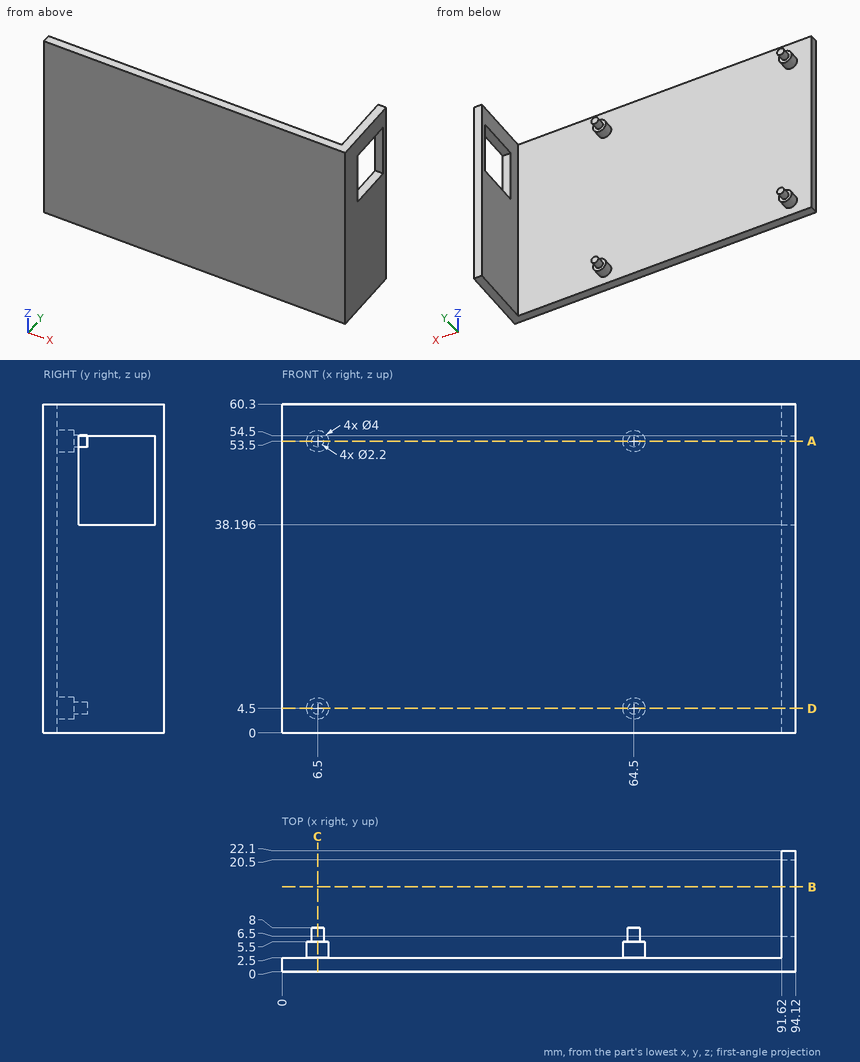
Geometry check sheet. Reference: drawing and pictorial views, mm from the part's lowest x, y, z. Coordinates: 2 decimals unless noted, no trailing zeros. Order: outer loops, then holes, each group sorted by start corner. A loop starts at its lowest first (then second) coordinate and runs counter-clockwise, first axis right, second up. Notation, with made-up numbers: (27, 78.5) - (42, 78.5) arc R18 ccw to (42, 98.5) - close; hole circle Ø8 at (73.5, -20.5). An arc over 180 degrees is marked (long way). Answer in a Markdown table with one row per item. Add a question column.
1) Cross-section at C-C, the plane x = 6.5. Record the cut outline in (y, z).
2) Material ranges on line 1 along Y through (x, z) = (12, 9.5); line 2 along X through (y, z) = (10.5, 20), recorded low to high. Write a range as [from, to].
3) Cross-section at D-D, the plane z = 4.5. Record the cut outline in (x, y).
4) Cross-section at B-B, the plane y = 15.5. Record the cut outline in (x, z), then the cut area to 3 significant figures.
5) Gauge pin test, flat ends, axial feed: P1, Ø6, axis at x = 52, z = 25.5, coming from the +Y side; P2, Ø1.8, axis at x = 64, z = 4.5, coming from the +Y side. Record the tip position at first contact, or that the pin passes through.
6) Cross-section at A-A, the plane z = 53.5. Record the cut outline in (x, y), then the cut area to 3 significant figures.
Check result:
| question | item | result |
|---|---|---|
| 1 | outline | (0, 0) - (2.5, 0) - (2.5, 2.5) - (5.5, 2.5) - (5.5, 3.4) - (8, 3.4) - (8, 5.6) - (5.5, 5.6) - (5.5, 6.5) - (2.5, 6.5) - (2.5, 51.5) - (5.5, 51.5) - (5.5, 52.4) - (8, 52.4) - (8, 54.6) - (5.5, 54.6) - (5.5, 55.5) - (2.5, 55.5) - (2.5, 60.3) - (0, 60.3) - close |
| 2 | line 1 | y = [0, 2.5] |
| 2 | line 2 | x = [91.62, 94.12] |
| 3 | outline | (0, 0) - (94.12, 0) - (94.12, 22.1) - (91.62, 22.1) - (91.62, 2.5) - (66.5, 2.5) - (66.5, 5.5) - (65.6, 5.5) - (65.6, 8) - (63.4, 8) - (63.4, 5.5) - (62.5, 5.5) - (62.5, 2.5) - (8.5, 2.5) - (8.5, 5.5) - (7.6, 5.5) - (7.6, 8) - (5.4, 8) - (5.4, 5.5) - (4.5, 5.5) - (4.5, 2.5) - (0, 2.5) - close |
| 4 | outline | (91.62, 0) - (94.12, 0) - (94.12, 38.2) - (91.62, 38.2) - close; (91.62, 54.5) - (94.12, 54.5) - (94.12, 60.3) - (91.62, 60.3) - close |
| 4 | area | 110 mm² |
| 5 | P1 | stops at y = 2.5 |
| 5 | P2 | stops at y = 8 |
| 6 | outline | (0, 0) - (94.12, 0) - (94.12, 6.5) - (91.62, 6.5) - (91.62, 2.5) - (66.5, 2.5) - (66.5, 5.5) - (65.6, 5.5) - (65.6, 8) - (63.4, 8) - (63.4, 5.5) - (62.5, 5.5) - (62.5, 2.5) - (8.5, 2.5) - (8.5, 5.5) - (7.6, 5.5) - (7.6, 8) - (5.4, 8) - (5.4, 5.5) - (4.5, 5.5) - (4.5, 2.5) - (0, 2.5) - close; (91.62, 20.5) - (94.12, 20.5) - (94.12, 22.1) - (91.62, 22.1) - close |
| 6 | area | 284 mm² |
